from build123d import *

# Parameters (mm, degrees)
SKETCH2_R           = 10.795
BOSS_EXTRUDE1_DEPTH = 12.7
SKETCH3_W           = 25.439299018
SKETCH3_H           = 7.62
CUT_EXTRUDE1_DEPTH  = 20.858349629
SKETCH5_R           = 1.27
CUT_EXTRUDE2_DEPTH  = 7.62


with BuildPart() as part:
    # Sketch2 → Boss-Extrude1 (new body)
    with BuildSketch(Plane(origin=(0, 0, 0), x_dir=(1, 0, 0), z_dir=(0, 1, 0))):
        with Locations(Location((0, 0, 0), (0, 0, 270))):
            Circle(SKETCH2_R)
    extrude(amount=-BOSS_EXTRUDE1_DEPTH)

    # Sketch3 → Cut-Extrude1 (cut, through all)
    with BuildSketch(Plane(origin=(0, 0, 0), x_dir=(0, 0, -1), z_dir=(1, 0, 0))):
        with Locations((-0.92844157, -6.35)):
            Rectangle(SKETCH3_W, SKETCH3_H)
    extrude(amount=CUT_EXTRUDE1_DEPTH, mode=Mode.SUBTRACT)

    # Sketch5 → Cut-Extrude2 (cut)
    with BuildSketch(Plane(origin=(0, 0, 0), x_dir=(1, 0, 0), z_dir=(0, 1, 0))):
        with Locations(Location((-4.318, -7.478995387, 0), (0, 0, 270))):
            Circle(SKETCH5_R)
        with Locations(Location((-4.318, 7.478995387, 0), (0, 0, 270))):
            Circle(SKETCH5_R)
    extrude(amount=-CUT_EXTRUDE2_DEPTH, mode=Mode.SUBTRACT)


solid = part.part
Source: CAD feature listing. Evaluate the final solid. Frame: model axes, mm. A direction names the side the tool comes from. Coordinates: 2 decimals unless noted, no trailing zeros. Loops run counter-clockwise (first coordinate to the right, second up) from the corner with the lowest first, then second, coordinate; pieces in that order, holes last. Notation, with made-up numbers: (-15, 17) -> (36, 17) arc R15 cw to (36, 45) -> close; hole circle Ø8 at (6.25, 15.25). An arc over 180 degrees is marked (long way). Answer in a Markdown table with one row per item. Add a question column.
Q1. Section B-B on z = 0. Return the cut outline in (x, y) (3 decimals), and give its area (3 significant figures).
Q2. Contact query for flat-ended pins moving along their axis: pin 1 Ø1.5 at (x, z) = (1.5, -2) entering from +Y; pin 2 Ø2 at (x, z) = (-4.5, 7.5) entering from +Y; pin 3 Ø4 at (y, z) = (-5, -4.5) entering from +X; pin 4 Ø5 at (x, y) = (-3.5, -2) entering from -Z. Output: stop coordinate, or through.
Q3. Reachability of faces 1 (the face through (0, 0, 0)), 2 (the face through (4, -10.16, 0)), 3 (the face through (-4.262, -3.757, -8.748)) from +Z, -Z, +X, -X, +Y, -Y: full face, straight path, thin tool, end or side. Return the list, or none.
Q4. Section D-D on x = 7.5. Return the cut outline in (y, z).
Q5. Section A-A on x = 0.5. Return the cut outline in (y, z).
Q6. Section C-C on y = -10.75. Return the cut outline in (x, z) (3 decimals), and give its area (3 significant figures).
Q7. Pull-direction query (Z, two-part tool) for faces 4 (the face through (4, -2.54, 0)), 5 (the face through (-9.577, -6.261, 4.981)), 6 (the face through (-4, -7.62, 7)); classes: pulls with the +Z half, pulls with the -Z half, needs draft (parallel to the pull), parting line crosses it, or undercut.
Q8. Ray query, line 1 along Y through (x, z) = (5.75, 5.25); line 2 along Z through (x, y) = (-4.75, -6.5); line 3 along Z through (x, y) = (-5.25, -2). Return the intervals inside material, ascending.
Computed values:
| question | item | result |
|---|---|---|
| 1 | outline | (-10.795, -12.7) -> (10.795, -12.7) -> (10.795, -10.16) -> (0, -10.16) -> (0, -2.54) -> (10.795, -2.54) -> (10.795, 0) -> (-10.795, 0) -> close |
| 1 | area | 192 mm^2 |
| 2 | pin 1 | stops at y = 0 |
| 2 | pin 2 | stops at y = -7.62 |
| 2 | pin 3 | stops at x = 0 |
| 2 | pin 4 | stops at z = -10.75 |
| 3 | face 1 | +Z, -Z, +X, -X, +Y |
| 3 | face 2 | +Z, -Z, +X |
| 3 | face 3 | +Y |
| 4 | outline | (-12.7, -7.76) -> (-10.16, -7.76) -> (-10.16, 7.76) -> (-12.7, 7.76) -> close; (-2.54, -7.76) -> (0, -7.76) -> (0, 7.76) -> (-2.54, 7.76) -> close |
| 5 | outline | (-12.7, -10.78) -> (-10.16, -10.78) -> (-10.16, 10.78) -> (-12.7, 10.78) -> close; (-2.54, -10.78) -> (0, -10.78) -> (0, 10.78) -> (-2.54, 10.78) -> close |
| 6 | outline | circle Ø21.59 at (0, 0) |
| 6 | area | 366 mm^2 |
| 7 | face 4 | needs draft |
| 7 | face 5 | parting line crosses it |
| 7 | face 6 | undercut |
| 8 | line 1 | y = -12.7 to -10.16, -2.54 to 0 |
| 8 | line 2 | z = -9.69 to -8.67, -6.28 to 6.28, 8.67 to 9.69 |
| 8 | line 3 | z = -9.43 to -8.34, -6.62 to 6.62, 8.34 to 9.43 |
